Read the model definition and answer for the solid it produces. Units are mm, in the model's axes. A direction names the side the tool comes from. Give positions to 0.01 mm unless a question says otherwise; leave off trailing zeros. Order: outer loops, then holes, each group sorted by start corner. A loop starts at its lowest first (then second) coordinate and runs counter-clockwise, first axis right, second up. Notation, with made-up numbers: M -30,43.5 L 26,43.5 A25 cw 26,67.5 Z; hole C 38,43 d6. An arc over 180 degrees is marked long. One line per item, written item: value.
from build123d import *

# Parameters (mm, degrees)
SKETCH1_R           = 4
SKETCH1_R_2         = 2.6
BOSS_EXTRUDE1_DEPTH = 9.8
CUT_EXTRUDE1_DEPTH  = 12.315476128
FILLET1_R           = 0.4


with BuildPart() as part:
    # Sketch1 → Boss-Extrude1 (new body)
    with BuildSketch(Plane(origin=(0, 0, 0), x_dir=(1, 0, 0), z_dir=(0, 1, 0))):
        with Locations(Location((0, 0, 0), (0, 0, 270))):
            Circle(SKETCH1_R)
        with Locations(Location((0, 0, 0), (0, 0, 270))):
            Circle(SKETCH1_R_2, mode=Mode.SUBTRACT)
    extrude(amount=BOSS_EXTRUDE1_DEPTH)

    # Sketch2 → Cut-Extrude1 (cut, through all)
    with BuildSketch(Plane(origin=(0, 9.8, 0), x_dir=(1, 0, 0), z_dir=(0, 1, 0))):
        with BuildLine():
            ThreePointArc((-1.838477631, 1.838477631), (-1.320191838, 2.737476443), (-1.322144063, 3.775173516))
            ThreePointArc((-1.322144063, 3.775173516), (0, 4), (1.322144063, 3.775173516))
            ThreePointArc((1.322144063, 3.775173516), (1.320191838, 2.737476443), (1.838477631, 1.838477631))
            ThreePointArc((1.838477631, 1.838477631), (0, 2.6), (-1.838477631, 1.838477631))
        make_face()
    extrude(amount=-CUT_EXTRUDE1_DEPTH, mode=Mode.SUBTRACT)

    # Fillet1
    fillet1_edges = [part.edges().sort_by_distance(p)[0] for p in [
        (-1.322144063, 4.9, -3.775173516),
        (1.322144063, 4.9, -3.775173516),
    ]]
    fillet(fillet1_edges, radius=FILLET1_R)


solid = part.part
1) Find section B-B, the plane x = 0. Write down the section's boundary in (y, z).
Reported:
outline: M 0,2.6 L 9.8,2.6 L 9.8,4 L 0,4 Z
2) Which of the six approach directions +Z, -Z, +X, -X, +Y, -Y give full straight-line access (tool end or side, diameter ignored) to faces 4 (the face through (-1.42, 4.97, -2.45)), 5 (the face through (0, 0, 3))?
Reported:
face 4: +Y, -Y
face 5: +Z, -Z, +X, -X, -Y
3) Find section C-C, the plane z = 1.25. Write down the section's boundary in (x, y), plus the area to 3 significant figures.
Reported:
outline: M -3.8,0 L -2.28,0 L -2.28,9.8 L -3.8,9.8 Z; M 2.28,0 L 3.8,0 L 3.8,9.8 L 2.28,9.8 Z
area: 29.8 mm^2
4) Determine the mould class of faces 1 (the face through (0, 5, 4)), 2 (the face through (0, 9.8, 3)), 3 (the face through (1.4, 5, -2.5)) for opening direction Z: +Z half, -Z half, draft (parallel to the pull), parting line (faces both ways), or undercut.
Reported:
face 1: parting line
face 2: draft
face 3: undercut
5) Find section D-D, the plane z = 3. Write down the section's boundary in (x, y).
Reported:
outline: M -2.65,0 L 2.65,0 L 2.65,9.8 L -2.65,9.8 Z
6) This flat-tipped pin is pushed along its axis until it touches: pin 1 Ø1 at (x, y) = (-1, 4) entering from -Z. Where does it stop, or does it pass through?
Reported:
pin 1: stops at z = -3.57
7) Find section A-A, the plane z = 0. Write down the section's boundary in (x, y), plus the area to 3 significant figures.
Reported:
outline: M -4,0 L -2.6,0 L -2.6,9.8 L -4,9.8 Z; M 2.6,0 L 4,0 L 4,9.8 L 2.6,9.8 Z
area: 27.4 mm^2
8) Consider probe 1 along X at (y, z) = (2.75, 0); probe 2 along Z at (x, y) = (0, 2.5); probe 3 along X at (y, z) = (7, -2). Determine where each line is inside the solid, lowest interval first.
Reported:
probe 1: x = -4 to -2.6, 2.6 to 4
probe 2: z = 2.6 to 4
probe 3: x = -3.46 to -1.69, 1.69 to 3.46
